```python
from build123d import *

# Parameters (mm, degrees)
SKETCH1_W           = 18
SKETCH1_H           = 55
BOSS_EXTRUDE1_DEPTH = 1
SKETCH2_W           = 7.6
SKETCH2_H           = 3.6
BOSS_EXTRUDE2_DEPTH = 1
SKETCH3_W           = 8
SKETCH3_H           = 3
CUT_EXTRUDE1_DEPTH  = 2
FILLET1_R           = 4


with BuildPart() as part:
    # Sketch1 → Boss-Extrude1 (new body)
    with BuildSketch(Plane(origin=(0, 0, 0), x_dir=(1, 0, 0), z_dir=(0, 1, 0))):
        with Locations((9, -27.5)):
            Rectangle(SKETCH1_W, SKETCH1_H)
    extrude(amount=BOSS_EXTRUDE1_DEPTH)

    # Sketch2 → Boss-Extrude2 (add)
    with BuildSketch(Plane.XZ):
        with Locations((9, 49)):
            Rectangle(SKETCH2_W, SKETCH2_H)
        with Locations((9, 39.6)):
            Rectangle(SKETCH2_W, SKETCH2_H)
    extrude(amount=BOSS_EXTRUDE2_DEPTH)

    # Sketch3 → Cut-Extrude1 (cut, through all)
    with BuildSketch(Plane.XZ):
        with Locations((9, 12.5)):
            Rectangle(SKETCH3_W, SKETCH3_H)
        with Locations((9, 6.5)):
            Rectangle(SKETCH3_W, SKETCH3_H)
        with Locations((9, 18.5)):
            Rectangle(SKETCH3_W, SKETCH3_H)
        with Locations((9, 24.5)):
            Rectangle(SKETCH3_W, SKETCH3_H)
    extrude(amount=-CUT_EXTRUDE1_DEPTH, mode=Mode.SUBTRACT)

    # Fillet1
    fillet1_edges = [part.edges().sort_by_distance(p)[0] for p in [
        (0, 0.5, 0),
        (18, 0.5, 0),
    ]]
    fillet(fillet1_edges, radius=FILLET1_R)


solid = part.part
```
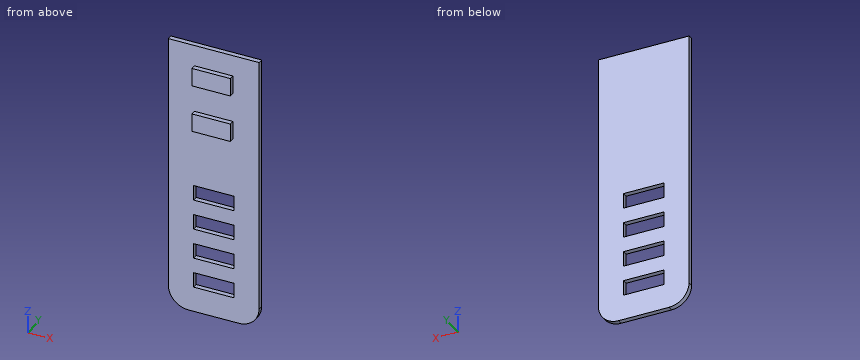
Source: CAD feature listing. Evaluate the final solid. Frame: model axes, mm. Coordinates: 2 decimals unless noted, no trailing zeros. Write each loop counter-clockwise with the first axis right and the second up, starting at its lowest first coordinate (ties: lowest second). Pieces come first, ordered by that corner, then holes. Notation, with made-up numbers: M 17,47 L 44,47 A13 cw 44,55 Z; hole C -20,27.25 d11. An arc over 180 degrees is marked long. Answer as a JSON object with one key per item and string values.
1. Cut plane A-A on y = 0.5. Output: boundary loops of the cut face in (x, z).
Evaluation:
{"outline": "M 0,4 A4 ccw 4,0 L 14,0 A4 ccw 18,4 L 18,55 L 0,55 Z; hole M 5,5 L 13,5 L 13,8 L 5,8 Z; hole M 5,11 L 13,11 L 13,14 L 5,14 Z; hole M 5,17 L 13,17 L 13,20 L 5,20 Z; hole M 5,23 L 13,23 L 13,26 L 5,26 Z"}
2. Ray query, L1, parallel to Z at x = 5.75, y = 0.4; L2, parallel to X at y = 0.2, z = 23.5; L3, parallel to Z at x = 6, y = -0.75. Return the intervals inside material, ascending.
Evaluation:
{"L1": "0 to 5, 8 to 11, 14 to 17, 20 to 23, 26 to 55", "L2": "0 to 5, 13 to 18", "L3": "37.8 to 41.4, 47.2 to 50.8"}
3. Cut plane B-B on x = 12. Output: boundary loops of the cut face in (y, z), plus the area to 3 significant figures.
Evaluation:
{"outline": "M -1,37.8 L 0,37.8 L 0,26 L 1,26 L 1,55 L 0,55 L 0,50.8 L -1,50.8 L -1,47.2 L 0,47.2 L 0,41.4 L -1,41.4 Z; M 0,0 L 1,0 L 1,5 L 0,5 Z; M 0,8 L 1,8 L 1,11 L 0,11 Z; M 0,14 L 1,14 L 1,17 L 0,17 Z; M 0,20 L 1,20 L 1,23 L 0,23 Z", "area": "50.2 mm^2"}
4. Cut plane D-D on x = 3.25. Output: boundary loops of the cut face in (y, z), plus the area to 3 significant figures.
Evaluation:
{"outline": "M 0,0.07 L 1,0.07 L 1,55 L 0,55 Z", "area": "54.9 mm^2"}
5. Cut plane C-C on z = 50. Output: boundary loops of the cut face in (x, y), plus the area to 3 significant figures.
Evaluation:
{"outline": "M 0,0 L 5.2,0 L 5.2,-1 L 12.8,-1 L 12.8,0 L 18,0 L 18,1 L 0,1 Z", "area": "25.6 mm^2"}
6. Contact query for flat-ended pins moving along their axis: P1, Ø6, axis at x = 13, z = 18, coming from the -Y side; P2, Ø1.1, axis at y = -0.5, z = 39, coming from the -X side; P3, Ø0.8, axis at y = -0.5, z = 49, coming from the -X side. Output: stop coordinate, or through.
Evaluation:
{"P1": "y = 0", "P2": "x = 0", "P3": "x = 5.2"}
